Check sheet for the modelled part. Datum: model origin and axes. Units: mm. Face numbers are marked on the shaded views. A direction names the side the tool comes from. Give positions to 0.01 mm unless a question says otherwise; leave off trailing zeros. Loops run counter-clockwise (first coordinate to the right, second up) from the corner with the lowest first, then second, coordinate; pieces in that order, holes last. Notation, with made-up numbers: (35, 0.25) -> (49, 0.25) arc R13 cw to (49, 24.25) -> close; hole circle Ø10 at (-22, 33.25). An arc over 180 degrees is marked (long way). Answer as CSV lines item,"result". Start each with the question number.
(1) Section check C-C on z = 7.5. Enter the section's corners in (x, y) (3 decimals), plus the area to 3 significant figures.
(2) Section check A-A on y = 0. Enter the section's corners in (x, z) (3 decimals).
(3) Gauge pin test, flat ends, axial feed: pin 1 Ø1 at (x, z) = (-1, 13.5) entering from +Y; pin 2 Ø2 at (x, z) = (1, 10.5) entering from +Y. Record the tip position at first contact, or that the pin passes through.
(4) Section check B-B on x = 0. Enter the section's corners in (y, z) (3 decimals), plus the area to 3 significant figures.
(5) Material ranges on line 1 (Z direction, x = -0.95, y = -1.7); line 2 (Y direction, x = -0.6, z = 12.5); line 3 (X direction, y = 0.65, z = 3.75), recorded low to high. Write a range as from..to.
(6) Access from +Z, -Z, +X, -X, +Y, -Y to the whole of each face (thin tool, end or side, straight path). Record for the marked faces 1 and 2.
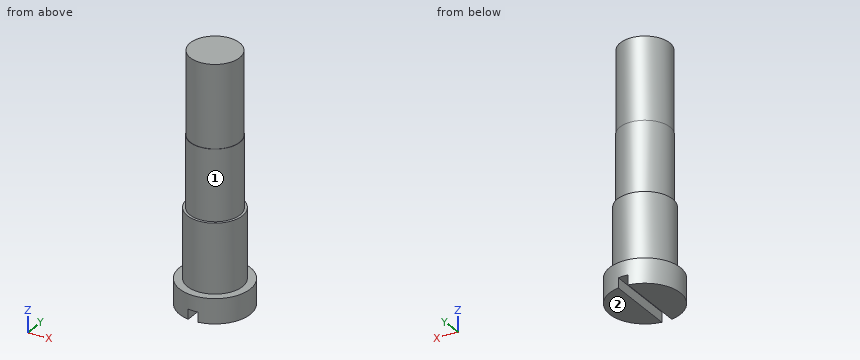
from build123d import *

# Parameters (mm, degrees)
F2_W          = 0.6
F2_H          = 0.6
F3_DEPTH      = 2.151
F3_DEPTH_BACK = 2.151


with BuildPart() as f1:
    # F0 (on Front) → F1 (revolve)
    with BuildSketch(Plane.XZ):
        Polygon((0, 15), (0, 0), (2.15, 0), (2.15, 1.5), (1.675, 1.5), (1.675, 5.7), (1.525, 5.7), (1.525, 10), (1.5, 10), (1.5, 15), align=None)
    revolve(axis=Axis((0, 0, 8.8781863451), (0, 0, -1)))

    # F2 (on Front) → F3 (cut, two sides)
    with BuildSketch(Plane.XZ) as f3_sk:
        with Locations((0, 0.3)):
            Rectangle(F2_W, F2_H)
    extrude(amount=-F3_DEPTH, mode=Mode.SUBTRACT)
    extrude(f3_sk.sketch, amount=F3_DEPTH_BACK, mode=Mode.SUBTRACT)


solid = f1.part
Working result:
1,outline,"circle Ø3.05 at (0, 0)"
1,area,"7.31 mm^2"
2,outline,"(-2.15, 0) -> (-0.3, 0) -> (-0.3, 0.6) -> (0.3, 0.6) -> (0.3, 0) -> (2.15, 0) -> (2.15, 1.5) -> (1.675, 1.5) -> (1.675, 5.7) -> (1.525, 5.7) -> (1.525, 10) -> (1.5, 10) -> (1.5, 15) -> (-1.5, 15) -> (-1.5, 10) -> (-1.525, 10) -> (-1.525, 5.7) -> (-1.675, 5.7) -> (-1.675, 1.5) -> (-2.15, 1.5) -> close"
3,pin 1,"stops at y = 1.41"
3,pin 2,"stops at y = 1.52"
4,outline,"(-2.15, 0.6) -> (2.15, 0.6) -> (2.15, 1.5) -> (1.675, 1.5) -> (1.675, 5.7) -> (1.525, 5.7) -> (1.525, 10) -> (1.5, 10) -> (1.5, 15) -> (-1.5, 15) -> (-1.5, 10) -> (-1.525, 10) -> (-1.525, 5.7) -> (-1.675, 5.7) -> (-1.675, 1.5) -> (-2.15, 1.5) -> close"
4,area,"46.1 mm^2"
5,line 1,"z = 0..1.5"
5,line 2,"y = -1.37..1.37"
5,line 3,"x = -1.54..1.54"
6,face 1,"+Z"
6,face 2,"-Z, +X, -X, +Y, -Y"
